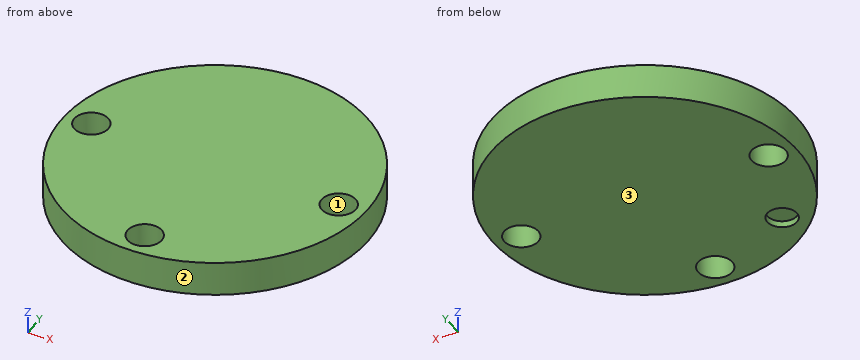
```python
from build123d import *

# Parameters (mm, degrees)
F0_W     = 47.5273691118
F0_H     = 10.7533988893
F2_R     = 5.3111422427
F3_DEPTH = 10.7543988893
F2_R_2   = 4.6185221062
F4_DEPTH = 2


with BuildPart() as f1:
    # F0 (on Front) → F1 (revolve)
    with BuildSketch(Plane.XZ):
        with Locations((-23.7636845559, -5.3766994447)):
            Rectangle(F0_W, F0_H)
    revolve(axis=Axis((0, 0, 11.207267642), (0, 0, 1)))

    # F2 (on face) → F3 (cut, through all)
    with BuildSketch(Plane(origin=(0, 0, -10.7533988893), x_dir=(1, 0, 0), z_dir=(0, 0, -1))):
        with Locations((-39.2993532375, 0)):
            Circle(F2_R)
        with Locations((0, 39.2993532375)):
            Circle(F2_R)
        with Locations((39.2993532375, 0)):
            Circle(F2_R)
    extrude(amount=-F3_DEPTH, mode=Mode.SUBTRACT)

    # F2 (on face) → F4 (cut)
    with BuildSketch(Plane(origin=(0, 0, -10.7533988893), x_dir=(1, 0, 0), z_dir=(0, 0, -1))):
        with Locations((-27.7888391705, 27.7888391705)):
            Circle(F2_R_2)
    extrude(amount=-F4_DEPTH, mode=Mode.SUBTRACT)


solid = f1.part
```
Can you work these out from the model? Positions are in its coordinate system, mm. Face numbers are marked on the shaded views. Round coordinates to 2 decimals unless told otherwise and drop trailing zeros. Loops run counter-clockwise (first coordinate to the right, second up) from the corner with the lowest first, then second, coordinate; pieces in that order, holes last. Notation, with made-up numbers: M 66.25,-2 L 84.25,-2 A20 ccw 84.25,30 Z; hole C -20.75,52.25 d1. An arc over 180 degrees is marked long. Answer as a JSON object with one key per item and string values. Group by question number.
Q1. Imagine slicing it at D-D, the plane z = -3.5. Please give me the cut outline in (x, y).
Q2. Imagine slicing it at C-C, the plane y = -37.5. Please give me the cut outline in (x, z), then the cut area to 3 significant figures.
Q3. Imagine slicing it at B-B, the plane x = 0. Please give me the cut outline in (y, z).
Q4. Will these pins go through, and if not, where does the flat tip stop? pin 1 (9.5 mm diameter, centred on x = 0, y = -39.3, fed in from +Z); pin 2 (3 mm diameter, centred on x = -17.5, z = -4.5, fed in from -Y); pin 3 (5 mm diameter, centred on x = 15, z = -2.5, fed in from -Y); pin 4 (2 mm diameter, centred on x = -28.5, z = -9, fed in from -Y).
Q5. Please list where these lines run through material, in increasing order: L1, parallel to X at y = 0, z = -2.25; L2, parallel to Y at x = 0, z = -6; L3, parallel to X at y = 3, z = -2.5.
Q6. Imagine slicing it at A-A, the plane y = 0. Please give me the cut outline in (x, z), then the cut area to 3 significant figures.
Q7. We'd pull the mould along X, two halves only. Please class the marked faces 1, 2 and 3: +X half, -X half, draft (parallel to the pull), parting line (faces both ways), or undercut.
Findings:
{
 "1": {"outline": "C 0,0 d95.05; hole C -39.3,0 d10.62; hole C 0,-39.3 d10.62; hole C 39.3,0 d10.62"},
 "2": {"outline": "M -29.2,-10.75 L -5,-10.75 L -5,0 L -29.2,0 Z; M 5,-10.75 L 29.2,-10.75 L 29.2,0 L 5,0 Z", "area": "521 mm2"},
 "3": {"outline": "M -47.53,-10.75 L -44.61,-10.75 L -44.61,0 L -47.53,0 Z; M -33.99,-10.75 L 47.53,-10.75 L 47.53,0 L -33.99,0 Z"},
 "4": {"pin 1": "passes through", "pin 2": "stops at y = -44.75", "pin 3": "stops at y = -45.85", "pin 4": "stops at y = -38.76"},
 "5": {"L1": "x = -47.53 to -44.61, -33.99 to 33.99, 44.61 to 47.53", "L2": "y = -47.53 to -44.61, -33.99 to 47.53", "L3": "x = -47.43 to -43.68, -34.92 to 34.92, 43.68 to 47.43"},
 "6": {"outline": "M -47.53,-10.75 L -44.61,-10.75 L -44.61,0 L -47.53,0 Z; M -33.99,-10.75 L 33.99,-10.75 L 33.99,0 L -33.99,0 Z; M 44.61,-10.75 L 47.53,-10.75 L 47.53,0 L 44.61,0 Z", "area": "794 mm2"},
 "7": {"face 1": "undercut", "face 2": "parting line", "face 3": "draft"}
}
